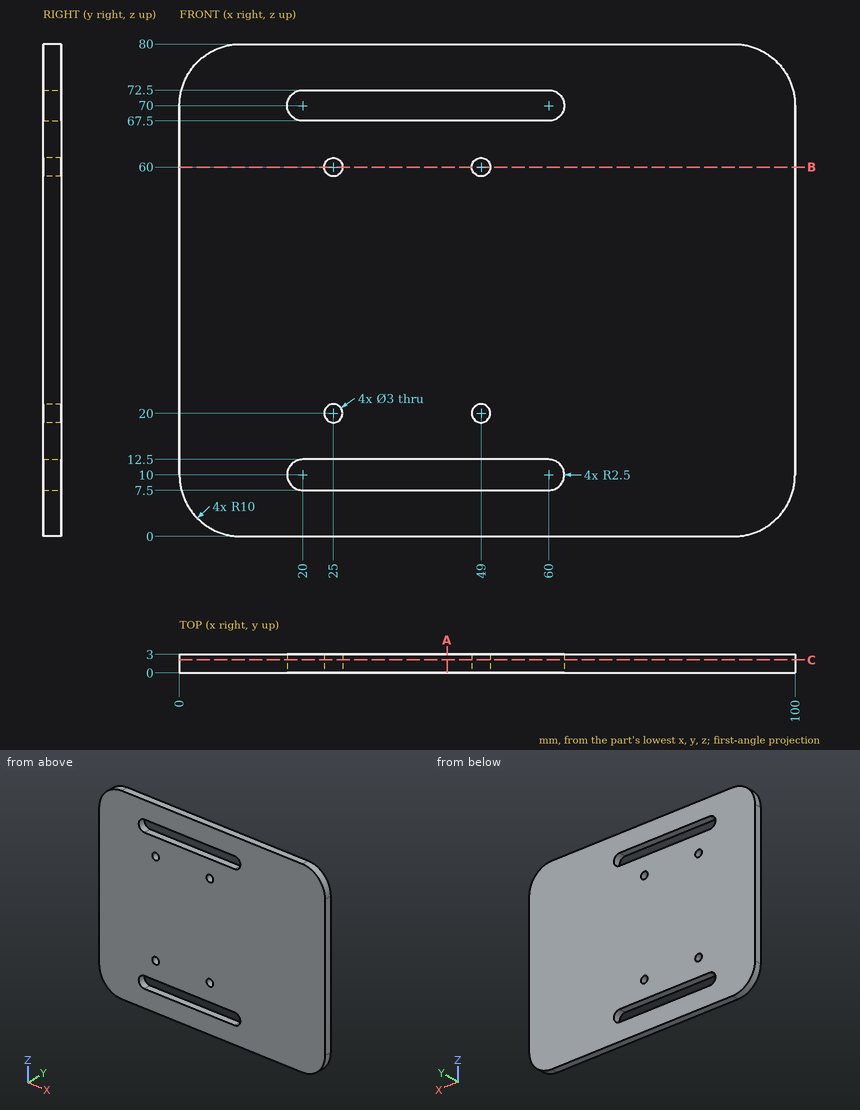
Job drawing, mm, ordinate dimensions from the low corner. One solid piece. Coordinates: 2 decimals unless noted, no trailing zeros. Order: outer loops, then holes, each group sorted by start corner. A loop starts at its lowest first (then second) coordinate and runs counter-clockwise, first axis right, second up. Notation, with made-up numbers: M 52.25,49.25 L 65.25,49.25 A25 ccw 65.25,86.25 Z; hole C 54,-21.75 d11. An arc over 180 degrees is marked long. Return JSON: item names as keys, results as strings.
1. Drill centre lines: probe 1 along X at (y, z) = (1.8, 20); probe 2 along Z at (x, y) = (59, 0.4); probe 3 along Z at (x, y) = (25, 1). Where is each one in solid material? Low to high.
Ans:
{"probe 1": "0 to 23.5, 26.5 to 47.5, 50.5 to 100", "probe 2": "0 to 7.5, 12.5 to 67.5, 72.5 to 80", "probe 3": "0 to 7.5, 12.5 to 18.5, 21.5 to 58.5, 61.5 to 67.5, 72.5 to 80"}
2. Flat gauge pins, fed straight in: pin 1 (2.5 mm diameter, centred on x = 25, z = 60, fed in from +Y); pin 2 (5 mm diameter, centred on x = 25, z = 20, fed in from +Y). Where does each tip first touch, or does it go through?
Ans:
{"pin 1": "through", "pin 2": "y = 3"}
3. Saw through at C-C (y = 2.1). Give the cut face in (x, z), and give its area (3 significant figures).
Ans:
{"outline": "M 0,10 A10 ccw 10,0 L 90,0 A10 ccw 100,10 L 100,70 A10 ccw 90,80 L 10,80 A10 ccw 0,70 Z; hole M 20,7.5 L 60,7.5 A2.5 ccw 60,12.5 L 20,12.5 A2.5 ccw Z; hole M 20,67.5 L 60,67.5 A2.5 ccw 60,72.5 L 20,72.5 A2.5 ccw Z; hole C 25,20 d3; hole C 25,60 d3; hole C 49,20 d3; hole C 49,60 d3", "area": "7,450 mm^2"}
4. Saw through at B-B (z = 60). Give the cut face in (x, y).
Ans:
{"outline": "M 0,0 L 23.5,0 L 23.5,3 L 0,3 Z; M 26.5,0 L 47.5,0 L 47.5,3 L 26.5,3 Z; M 50.5,0 L 100,0 L 100,3 L 50.5,3 Z"}
5. Saw through at A-A (x = 43.5). Give the cut face in (y, z), and give its area (3 significant figures).
Ans:
{"outline": "M 0,0 L 3,0 L 3,7.5 L 0,7.5 Z; M 0,12.5 L 3,12.5 L 3,67.5 L 0,67.5 Z; M 0,72.5 L 3,72.5 L 3,80 L 0,80 Z", "area": "210 mm^2"}
